```python
from build123d import *

# Parameters (mm, degrees)
SKETCH1_R           = 31.65
BOSS_EXTRUDE1_DEPTH = 5
CHAMFER1_SIZE       = 0.5
SKETCH2_R           = 11.2
BOSS_EXTRUDE2_DEPTH = 8
SKETCH3_R           = 16
BOSS_EXTRUDE3_DEPTH = 38
SKETCH5_R           = 9.5
CUT_EXTRUDE2_DEPTH  = 52
CUT_EXTRUDE3_REACH  = 53
SKETCH6_R           = 2
SKETCH6_R_2         = 4
SKETCH8_OUTSIDE_W   = 85.906
SKETCH8_OUTSIDE_H   = 85.906
SKETCH8_OUTSIDE_R   = 31.15
SKETCH8_OUTSIDE_R_2 = 4
CUT_EXTRUDE4_DEPTH  = 10


with BuildPart() as part:
    # Sketch1 → Boss-Extrude1 (new body)
    with BuildSketch(Plane.XY):
        Circle(SKETCH1_R)
    extrude(amount=BOSS_EXTRUDE1_DEPTH)

    # Chamfer1
    chamfer1_edges = [part.edges().sort_by_distance(p)[0] for p in [
        (-31.65, 0, 0),
        (-31.65, 0, 5),
    ]]
    chamfer(chamfer1_edges, length=CHAMFER1_SIZE)

    # Sketch2 → Boss-Extrude2 (add)
    with BuildSketch(Plane.XY.offset(5)):
        Circle(SKETCH2_R)
    extrude(amount=BOSS_EXTRUDE2_DEPTH)

    # Sketch3 → Boss-Extrude3 (add)
    with BuildSketch(Plane.XY.offset(13)):
        Circle(SKETCH3_R)
    extrude(amount=BOSS_EXTRUDE3_DEPTH)

    # Sketch5 → Cut-Extrude2 (cut, through all)
    with BuildSketch(Plane(origin=(0, 0, 0), x_dir=(-1, 0, 0), z_dir=(0, 0, -1))):
        Circle(SKETCH5_R)
    extrude(amount=-CUT_EXTRUDE2_DEPTH, mode=Mode.SUBTRACT)

    # Sketch6 → Cut-Extrude3 (cut, up to next)
    with BuildSketch(Plane(origin=(0, 0, 0), x_dir=(-1, 0, 0), z_dir=(0, 0, -1)), mode=Mode.PRIVATE) as cut_extrude3_sk1:
        with Locations((21.35, 9.9)):
            Circle(SKETCH6_R)
    cut_extrude3_tool1 = extrude(cut_extrude3_sk1.sketch, amount=-CUT_EXTRUDE3_REACH, mode=Mode.PRIVATE) & part.part
    add(cut_extrude3_tool1.solids().sort_by_distance((-21.35, 9.9, 0))[0], mode=Mode.SUBTRACT)
    # Sketch6 → Cut-Extrude3 (cut, up to next)
    with BuildSketch(Plane(origin=(0, 0, 0), x_dir=(-1, 0, 0), z_dir=(0, 0, -1)), mode=Mode.PRIVATE) as cut_extrude3_sk2:
        with Locations((-21.35, 9.9)):
            Circle(SKETCH6_R)
    cut_extrude3_tool2 = extrude(cut_extrude3_sk2.sketch, amount=-CUT_EXTRUDE3_REACH, mode=Mode.PRIVATE) & part.part
    add(cut_extrude3_tool2.solids().sort_by_distance((21.35, 9.9, 0))[0], mode=Mode.SUBTRACT)
    # Sketch6 → Cut-Extrude3 (cut, up to next)
    with BuildSketch(Plane(origin=(0, 0, 0), x_dir=(-1, 0, 0), z_dir=(0, 0, -1)), mode=Mode.PRIVATE) as cut_extrude3_sk3:
        with Locations((-21.35, -9.9)):
            Circle(SKETCH6_R)
    cut_extrude3_tool3 = extrude(cut_extrude3_sk3.sketch, amount=-CUT_EXTRUDE3_REACH, mode=Mode.PRIVATE) & part.part
    add(cut_extrude3_tool3.solids().sort_by_distance((21.35, -9.9, 0))[0], mode=Mode.SUBTRACT)
    # Sketch6 → Cut-Extrude3 (cut, up to next)
    with BuildSketch(Plane(origin=(0, 0, 0), x_dir=(-1, 0, 0), z_dir=(0, 0, -1)), mode=Mode.PRIVATE) as cut_extrude3_sk4:
        with Locations((21.35, -9.9)):
            Circle(SKETCH6_R)
    cut_extrude3_tool4 = extrude(cut_extrude3_sk4.sketch, amount=-CUT_EXTRUDE3_REACH, mode=Mode.PRIVATE) & part.part
    add(cut_extrude3_tool4.solids().sort_by_distance((-21.35, -9.9, 0))[0], mode=Mode.SUBTRACT)
    # Sketch6 → Cut-Extrude3 (cut, up to next)
    with BuildSketch(Plane(origin=(0, 0, 0), x_dir=(-1, 0, 0), z_dir=(0, 0, -1)), mode=Mode.PRIVATE) as cut_extrude3_sk5:
        with Locations((11.648195828, -19.6)):
            Circle(SKETCH6_R_2)
    cut_extrude3_tool5 = extrude(cut_extrude3_sk5.sketch, amount=-CUT_EXTRUDE3_REACH, mode=Mode.PRIVATE) & part.part
    add(cut_extrude3_tool5.solids().sort_by_distance((-11.648196, -19.6, 0))[0], mode=Mode.SUBTRACT)
    # Sketch6 → Cut-Extrude3 (cut, up to next)
    with BuildSketch(Plane(origin=(0, 0, 0), x_dir=(-1, 0, 0), z_dir=(0, 0, -1)), mode=Mode.PRIVATE) as cut_extrude3_sk6:
        with Locations((-8.732486564, 15.622964243)):
            Circle(SKETCH6_R)
    cut_extrude3_tool6 = extrude(cut_extrude3_sk6.sketch, amount=-CUT_EXTRUDE3_REACH, mode=Mode.PRIVATE) & part.part
    add(cut_extrude3_tool6.solids().sort_by_distance((8.732487, 15.622964, 0))[0], mode=Mode.SUBTRACT)
    # Sketch6 → Cut-Extrude3 (cut, up to next)
    with BuildSketch(Plane(origin=(0, 0, 0), x_dir=(-1, 0, 0), z_dir=(0, 0, -1)), mode=Mode.PRIVATE) as cut_extrude3_sk7:
        with Locations((-9.163640635, -15.374037324)):
            Circle(SKETCH6_R)
    cut_extrude3_tool7 = extrude(cut_extrude3_sk7.sketch, amount=-CUT_EXTRUDE3_REACH, mode=Mode.PRIVATE) & part.part
    add(cut_extrude3_tool7.solids().sort_by_distance((9.163641, -15.374037, 0))[0], mode=Mode.SUBTRACT)
    # Sketch6 → Cut-Extrude3 (cut, up to next)
    with BuildSketch(Plane(origin=(0, 0, 0), x_dir=(-1, 0, 0), z_dir=(0, 0, -1)), mode=Mode.PRIVATE) as cut_extrude3_sk8:
        with Locations((17.896127199, -0.248926919)):
            Circle(SKETCH6_R)
    cut_extrude3_tool8 = extrude(cut_extrude3_sk8.sketch, amount=-CUT_EXTRUDE3_REACH, mode=Mode.PRIVATE) & part.part
    add(cut_extrude3_tool8.solids().sort_by_distance((-17.896127, -0.248927, 0))[0], mode=Mode.SUBTRACT)

    # Sketch7 → Cut-Revolve3 (revolve, cut)
    with BuildSketch(Plane(origin=(0, 0, 0), x_dir=(1, 0, 0), z_dir=(0, 1, 0))):
        with BuildLine():
            Line((-8.5, -42.6), (-8.5, -46.6))
            ThreePointArc((-8.5, -46.6), (-10.5, -44.6), (-8.5, -42.6))
        make_face()
    revolve(axis=Axis((0, 0, 44.6), (0, 0, 1)), mode=Mode.SUBTRACT)

    # Sketch8 outside → Cut-Extrude4 (cut)
    with BuildSketch(Plane(origin=(0, 0, 0), x_dir=(-1, 0, 0), z_dir=(0, 0, -1))):
        Rectangle(SKETCH8_OUTSIDE_W, SKETCH8_OUTSIDE_H)
        Circle(SKETCH8_OUTSIDE_R, mode=Mode.SUBTRACT)
        with Locations((-22.798195828, -0.287633496)):
            Circle(SKETCH8_OUTSIDE_R_2)
        with Locations((11.15, 19.887633496)):
            Circle(SKETCH8_OUTSIDE_R_2)
    extrude(amount=-CUT_EXTRUDE4_DEPTH, mode=Mode.SUBTRACT)


solid = part.part
```
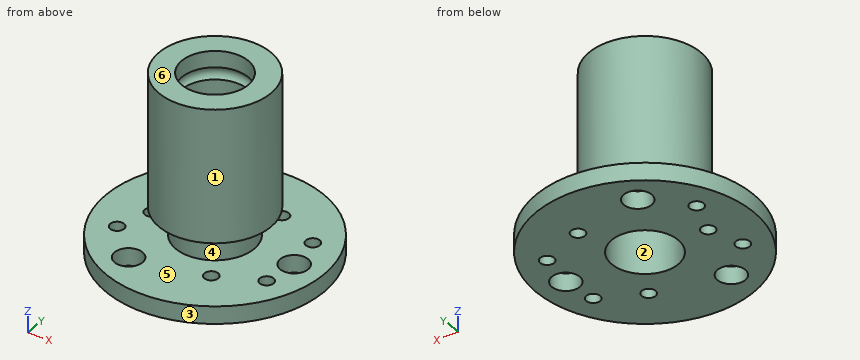
Part model, mm, in its own coordinate system. Face numbers are marked on the shaded views. A direction names the side the tool comes from. Round coordinates to 2 decimals unless told otherwise and drop trailing zeros. Write each loop counter-clockwise with the first axis right and the second up, starting at its lowest first coordinate (ties: lowest second). Pieces come first, ordered by that corner, then holes. Notation, with made-up numbers: (60, 13) -> (72, 13) arc R20 cw to (72, 46) -> close; hole circle Ø11 at (26, 21). An arc over 180 degrees is marked (long way). Return JSON: item names as keys, results as strings. Group by question number.
Q1. Probe L1, parallel to Y at x = 0, z = 34; L2, parallel to Z at x = 27, y = -11.5; L3, parallel to Z at x = 4.5, y = 11. List the from-to ranges inside material, lowest first. Write a range as [from, to].
Q2. Pin check, flat tips, straight feed: pin 1 (2 mm diameter, centred on y = 4, z = 34, fed in from +X); pin 2 (6.5 mm diameter, centred on x = -21.35, y = -9.9, fed in from +Z); pin 3 (12 mm diameter, centred on x = 15.5, z = 30.5, fed in from +Y). Stop position of each tip, or through.
Q3. Which spindle directions (+Z, -Z, +X, -X, +Y, -Y) get a long thin tool onto all of the face, cutting with end or side? Do the marked faces 1 and 2. Say none if no direction does.
Q4. Saw through at A-A on x = 0. Write the cut outline in (y, z), plus the area to 3 significant figures.
Q5. Saw through at C-C on z = 34. Write the cut outline in (x, y).
Q6. Saw through at B-B on x = 22. Write the cut outline in (y, z).
Q7. Mould opens along Z. For the marked faces 3, 4, 5 and 6 say: pulls with the +Z half, pulls with the -Z half, needs draft (parallel to the pull), parting line crosses it, or undercut.
Q8. Saw through at D-D on x = -21.35. Write the cut outline in (y, z), plus the area to 3 significant figures.
Answer:
{
 "1": {"L1": "[-16, -9.5], [9.5, 16]", "L2": "[0, 5]", "L3": "[0, 5], [13, 51]"},
 "2": {"pin 1": "x = 15.72", "pin 2": "z = 5", "pin 3": "y = 12.87"},
 "3": {"face 1": "+Z", "face 2": "+Z, -Z"},
 "4": {"outline": "(-31.15, 0) -> (-9.5, 0) -> (-9.5, 42.87) arc R2 cw to (-9.5, 46.33) -> (-9.5, 51) -> (-16, 51) -> (-16, 13) -> (-11.2, 13) -> (-11.2, 5) -> (-31.15, 5) -> close; (9.5, 0) -> (31.15, 0) -> (31.15, 5) -> (11.2, 5) -> (11.2, 13) -> (16, 13) -> (16, 51) -> (9.5, 51) -> (9.5, 46.33) arc R2 cw to (9.5, 42.87) -> close", "area": "733 mm2"},
 "5": {"outline": "circle Ø32 at (0, 0); hole circle Ø19 at (0, 0)"},
 "6": {"outline": "(-22.05, 0) -> (-11.79, 0) -> (-11.79, 5) -> (-22.05, 5) -> close; (-8.01, 0) -> (-4.21, 0) -> (-4.21, 5) -> (-8.01, 5) -> close; (3.63, 0) -> (8.01, 0) -> (8.01, 5) -> (3.63, 5) -> close; (11.79, 0) -> (22.05, 0) -> (22.05, 5) -> (11.79, 5) -> close"},
 "7": {"face 3": "needs draft", "face 4": "undercut", "face 5": "undercut", "face 6": "pulls with the +Z half"},
 "8": {"outline": "(-22.68, 0) -> (-11.9, 0) -> (-11.9, 5) -> (-22.68, 5) -> close; (-7.9, 0) -> (7.9, 0) -> (7.9, 5) -> (-7.9, 5) -> close; (11.9, 0) -> (22.68, 0) -> (22.68, 5) -> (11.9, 5) -> close", "area": "187 mm2"}
}
